from build123d import *

# Parameters (mm, degrees)
SKETCH_1_R          = 45
SKETCH_1_R_2        = 32
EXTRUDE_1_DEPTH     = 30
SKETCH_2_R          = 2.4455
CUT_EXTRUDE_1_DEPTH = 18
CHAMFER_1_SIZE      = 0.5545


with BuildPart() as part:
    # Эскиз1 → Бобышка-Вытянуть1 (new body)
    with BuildSketch(Plane.XY):
        Circle(SKETCH_1_R)
        Circle(SKETCH_1_R_2, mode=Mode.SUBTRACT)
    extrude(amount=EXTRUDE_1_DEPTH)

    # Эскиз2 → Вырез-Вытянуть1 (cut)
    with BuildSketch(Plane(origin=(0, 0, 0), x_dir=(-1, 0, 0), z_dir=(0, 0, -1))):
        with Locations((0, 45)):
            Circle(SKETCH_2_R)
    extrude(amount=-CUT_EXTRUDE_1_DEPTH, mode=Mode.SUBTRACT)

    # Фаска1
    chamfer_1_edges = [part.edges().sort_by_distance(p)[0] for p in [
        (0, 42.5545, 0),
    ]]
    chamfer(chamfer_1_edges, length=CHAMFER_1_SIZE)


solid = part.part
Can you work these out from the model? Positions are in its coordinate system, mm. A direction names the side the tool comes from. Coordinates: 2 decimals unless noted, no trailing zeros. Loops run counter-clockwise (first coordinate to the right, second up) from the corner with the lowest first, then second, coordinate; pieces in that order, holes last. Notation, with made-up numbers: (-22, 1.5) - (4, 1.5) arc R15 ccw to (4, 11.5) - close; hole circle Ø4 at (79.5, 6). An arc over 180 degrees is marked (long way). Answer as a JSON object with one key per item and string values. Group by question number.
Item 1: On a 3-axis mill with a long thin cutter (end or side, diameter ignored), from which of +Z, -Z, +X, -X, +Y, -Y can I reach the whole of each face in a straight line? I mean faces 1 (the face through (0.053, 42.555, 9.155)), 2 (the face through (-6.94, -31.24, 14.79)). Say none if no direction works.
Item 2: If we section it at C-C (z = 20.5): List the corners of the cut face in (x, y) for me, plus the area to 3 significant figures.
Item 3: If I drill on L1, parallel to Y at x = 0, z = 21.75; L2, parallel to Y at x = 0, z = 14; L3, parallel to X at y = -1.5, z = 15 (3 decimals), over which ranges is the centre line in solid material (lowest first)? Write a range as from..to.
Item 4: If we section it at B-B (x = 0): List the corners of the cut face in (y, z) for me.
Item 5: If we section it at D-D (x = 29): List the corners of the cut face in (y, z) for me, plus the area to 3 significant figures.
Item 6: For pin 1 (4 mm diameter, centred on x = -24, z = 11, fed in from +Y); pin 2 (2.5 mm diameter, centred on x = 0.5, y = 43.5, fed in from -Z); pin 3 (5 mm diameter, centred on y = 19.5, z = 11.5, fed in from -X), each with a flat end and sliding along its axis, tell me the tip position at first contact or that it passes through.
Item 7: If we mould it in two halves opening along X, with no side actions, what happens to faces 3 (the face through (20.765, -39.923, 14.79)), 4 (the face through (0.1, 42.4, 0.4)), 5 (the face through (-11, 31, 0))? For each: released by +X, released by -X, zero draft, split by the parting line, or undercut.
Item 8: If we section it at A-A (y = 0): List the corners of the cut face in (x, z) for me, plus the area to 3 significant figures.
Returned:
{
 "1": {"face 1": "-Z, +Y", "face 2": "+Z, -Z"},
 "2": {"outline": "circle Ø90 at (0, 0); hole circle Ø64 at (0, 0)", "area": "3,140 mm²"},
 "3": {"L1": "y = -45..-32, 32..45", "L2": "y = -45..-32, 32..42.55", "L3": "x = -44.975..-31.965, 31.965..44.975"},
 "4": {"outline": "(-45, 0) - (-32, 0) - (-32, 30) - (-45, 30) - close; (32, 0) - (42, 0) - (42.55, 0.55) - (42.55, 18) - (45, 18) - (45, 30) - (32, 30) - close"},
 "5": {"outline": "(-34.41, 0) - (-13.53, 0) - (-13.53, 30) - (-34.41, 30) - close; (13.53, 0) - (34.41, 0) - (34.41, 30) - (13.53, 30) - close", "area": "1,250 mm²"},
 "6": {"pin 1": "stops at y = 39.26", "pin 2": "stops at z = 0.17", "pin 3": "stops at x = -41.67"},
 "7": {"face 3": "split by the parting line", "face 4": "undercut", "face 5": "zero draft"},
 "8": {"outline": "(-45, 0) - (-32, 0) - (-32, 30) - (-45, 30) - close; (32, 0) - (45, 0) - (45, 30) - (32, 30) - close", "area": "780 mm²"}
}
